Autodesk Inventor part; units mm, degrees
ref_plane "YZ Plane" through (0, 0, 0) normal (1, 0, 0) x (0, 1, 0)
ref_plane "XZ Plane" through (0, 0, 0) normal (0, 1, 0) x (-1, 0, 0)
ref_plane "XY Plane" through (0, 0, 0) normal (0, 0, 1) x (1, 0, 0)
sketch "Sketch1" plane through (0, 0, 0) normal (0, 0, 1) x (1, 0, 0)
  line L0 (9.75, 13) -> (7.875, 9.7524)
  line L1 (7.875, 9.7524) -> (4.125, 9.7524)
  line L2 (4.125, 9.7524) -> (2.25, 13)
  line L3 (2.25, 13) -> (4.125, 16.2476)
  line L4 (4.125, 16.2476) -> (7.875, 16.2476)
  line L5 (7.875, 16.2476) -> (9.75, 13)
  point P0 (0, 0)
  point P1 (6, 13)
  dimension "d0" = 7.5
extrude "Extrusion1" add sketch "Sketch1" along normal blind 18
sketch "Sketch2" plane through (4.125, 16.2476, 0) normal (0, 1, 0) x (1, 0, 0)
  line L0 (3.75, -18) -> (5.625, -18)
  line L1 (3.75, -18) -> (0, -18)
  line L2 (0, -18) -> (-6.6597, -33.0128)
  line L3 (-1.875, 0) -> (-1.875, -18)
  line L4 (-6.6597, -45.8247) -> (-6.6597, -33.0128)
  line L5 (3.75, -18) -> (1.875, -18)
  line L6 (9.3403, -45.8668) -> (9.3403, -32.8539)
  line L7 (9.3403, -32.8539) -> (3.75, -18)
  line L8 (9.3403, -45.8668) -> (7.3403, -45.8668)
  line L9 (7.3403, -45.8668) -> (7.3403, -33.2178)
  line L10 (-6.6597, -45.8247) -> (-4.6597, -45.8247)
  line L11 (-4.6597, -45.8247) -> (-4.6597, -33.4364)
  line L12 (2.1735, -18.0436) -> (2.158, -18)
  line L13 (1.875, -29) -> (5.7529, -29)
  line L14 (-2.6917, -29) -> (1.875, -29)
  line L15 (-4.6597, -33.4364) -> (-2.6917, -29)
  line L16 (5.7529, -29) -> (7.3403, -33.2178)
  line L17 (1.875, -18) -> (1.875, -45.8247)
  point P0 (-4.125, 0)
  dimension "d12" = 2
  dimension "d13" = 2
  dimension "d16" = 27.8247
  dimension "d17" = 11
  dimension "d21" = 12
  dimension "d31" = 2
  dimension "d32" = 2
extrude "Extrusion2" add sketch "Sketch2" against normal blind 6.5
sketch "Sketch3" plane through (-2.5347, 9.7476, 33.0128) normal (-0.9141, 0, -0.4055) x (-0.4055, 0, 0.9141)
  point P0 (-31.2047, -9.7476)
sketch "Sketch5" plane through (4.125, 16.2476, 0) normal (0, 1, 0) x (1, 0, 0)
  line L0 (-1.875, -18) -> (0, -18)
  line L1 (-1.875, -18) -> (-1.875, -22.2268)
  line L2 (0, -18) -> (-6.6597, -33.0128)
  line L3 (3.75, -18) -> (5.625, -18)
  line L4 (5.625, -18) -> (5.625, -22.982)
  line L5 (9.3403, -32.8539) -> (3.75, -18)
  point P0 (-4.125, 0)
extrude "Extrusion3" add sketch "Sketch5" against normal blind 6.5
sketch "Sketch6" plane through (13.4653, 16.2476, 45.8668) normal (1, 0, 0) x (0, 0, -1)
  line L0 (0, 0) -> (0, -3.25)
  line L1 (0, 0) -> (0, -6.5)
  line L2 (0, -3.25) -> (6, -3.25)
  circle A0 centre (6, -3.25) radius 1.5
  point P0 (45.8668, -16.2476)
  dimension "d27" = 6
  dimension "d28" = 3
extrude "Extrusion4" cut sketch "Sketch6" against normal through all
properties part number "Test de pincev2"
Design review of the part built by this model. Coordinates are the model's own, in mm. A direction names the side the tool comes from. Give positions to 0.01 mm unless a question says otherwise; leave off trailing zeros. Order: outer loops, then holes, each group sorted by start corner. A loop starts at its lowest first (then second) coordinate and runs counter-clockwise, first axis right, second up. Notation, with made-up numbers: (-16.5, -32.75) - (33.5, -32.75) arc R25 cw to (33.5, -11.75) - close; hole circle Ø9 at (-6, -5.75). An arc over 180 degrees is marked (long way). Use CSV: the item, a comma, the result in double quotes. Start each with the question number.
Q1. Take a section at B-B (y = 13.5). State the section outline as (x, z) points.
Q2. Draft analysis for pull direction X (two halves, no side actions). For faces 1 (the face through (10.66, 13.04, 31.08)), 2 (the face through (5.4, 9.748, 28.6)), 3 (the face through (11.634, 13.043, 27.987)), state which applies: pulls with the +X half, pulls with the -X half, needs draft (parallel to the pull), parting line crosses it, or undercut.
Q3. For line 1 (X direction, y = 15.75, z = 33.5); line 2 (Z direction, x = 2.75, y = 11); line 3 (X direction, y = 12.25, z = 32), list the stretches that pass through material, from the lowest coordinate up.
Q4. For P1, Ø2, axis at x = 3.5, y = 13.5, coming from the +Z side; P2, Ø1.9, axis at x = 5.5, z = 5, coming from the -Y side; P3, Ø1, axis at x = -1, y = 14.5, coming from the +Z side; P4, Ø2.5, axis at x = 4.5, y = 11.5, coming from the -Z side, all flat-tipped, find the tip position at first contact; note any pin that passes through.
Q5. Take a section at A-A (z = 43). State the section outline as (x, y) points.
Q6. Machinability: for faces 4 (the face through (3.174, 14.601, 8.874)), 5 (the face through (0.436, 13.043, 31.249)), 6 (the face through (8.826, 11.399, 8.874)), which of the approach directions +Z, -Z, +X, -X, +Y, -Y give a long, thin tool a straight path to every point of the face, cutting with its end or side? Answer none if there is none.
Q7. Take a section at C-C (z = 15). State the section outline as (x, y) points (3 decimals).
Q8. Take a section at D-D (y = 15.25). State the section outline as (x, z) points.
Calculated:
1,outline,"(-2.53, 33.01) - (2.25, 22.23) - (2.25, 18) - (2.54, 18) - (2.54, 0) - (9.46, 0) - (9.46, 18) - (9.75, 18) - (9.75, 22.98) - (13.47, 32.85) - (13.47, 38.45) - (11.47, 38.45) - (11.47, 33.22) - (9.88, 29) - (1.43, 29) - (-0.53, 33.44) - (-0.53, 38.45) - (-2.53, 38.45) - close; (-2.53, 41.28) - (-0.53, 41.28) - (-0.53, 45.82) - (-2.53, 45.82) - close; (11.47, 41.28) - (13.47, 41.28) - (13.47, 45.87) - (11.47, 45.87) - close"
2,face 1,"undercut"
2,face 2,"needs draft"
2,face 3,"pulls with the +X half"
3,line 1,"x = -2.53 to -0.53, 11.47 to 13.47"
3,line 2,"z = 18 to 29"
3,line 3,"x = -2.09 to 0.1, 11.01 to 13.14"
4,P1,"stops at z = 29"
4,P2,"stops at y = 9.75"
4,P3,"stops at z = 45.82"
4,P4,"stops at z = 0"
5,outline,"(-2.53, 9.75) - (-0.53, 9.75) - (-0.53, 16.25) - (-2.53, 16.25) - close; (11.47, 9.75) - (13.47, 9.75) - (13.47, 16.25) - (11.47, 16.25) - close"
6,face 4,"-Z, -X, +Y"
6,face 5,"+Z, +Y, -Y"
6,face 6,"-Z, +X, -Y"
7,outline,"(2.25, 13) - (4.125, 9.752) - (7.875, 9.752) - (9.75, 13) - (7.875, 16.248) - (4.125, 16.248) - close"
8,outline,"(-2.53, 33.01) - (2.25, 22.23) - (2.25, 18) - (3.55, 18) - (3.55, 0) - (8.45, 0) - (8.45, 18) - (9.75, 18) - (9.75, 22.98) - (13.47, 32.85) - (13.47, 45.87) - (11.47, 45.87) - (11.47, 33.22) - (9.88, 29) - (1.43, 29) - (-0.53, 33.44) - (-0.53, 45.82) - (-2.53, 45.82) - close"
